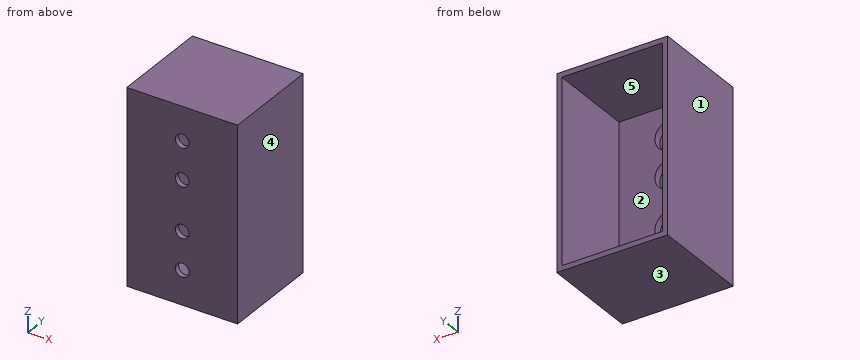
from build123d import *

# Parameters (mm, degrees)
EXTRUDE_1_DEPTH     = 73
SKETCH_2_W          = 44
SKETCH_2_H          = 39.5
EXTRUDE_2_DEPTH     = 2
SKETCH_3_W          = 44
SKETCH_3_H          = 39.5
EXTRUDE_3_DEPTH     = 2
SKETCH_4_R          = 2.75
CUT_EXTRUDE_1_DEPTH = 10
SKETCH_5_R          = 5.75
SKETCH_5_R_2        = 2.75
CUT_EXTRUDE_2_DEPTH = 3


with BuildPart() as part:
    # 草图1 → 凸台-拉伸1 (new body)
    with BuildSketch(Plane.XY):
        Polygon((-17.828125, 6.526041667), (-17.828125, -32.973958333), (26.171875, -32.973958333), (26.171875, 6.526041667), (24.171875, 6.526041667), (24.171875, -27.973958333), (-15.828125, -27.973958333), (-15.828125, 6.526041667), align=None)
    extrude(amount=EXTRUDE_1_DEPTH)

    # 草图2 → 凸台-拉伸2 (add)
    with BuildSketch(Plane.XY.offset(73)):
        with Locations((4.171875, -13.223958333)):
            Rectangle(SKETCH_2_W, SKETCH_2_H)
    extrude(amount=EXTRUDE_2_DEPTH)

    # 草图3 → 凸台-拉伸3 (add)
    with BuildSketch(Plane(origin=(0, 0, 0), x_dir=(-1, 0, 0), z_dir=(0, 0, -1))):
        with Locations((-4.171875, -13.223958333)):
            Rectangle(SKETCH_3_W, SKETCH_3_H)
    extrude(amount=EXTRUDE_3_DEPTH)

    # 草图4 → 切除-拉伸1 (cut)
    with BuildSketch(Plane(origin=(0, -27.973958333, 0), x_dir=(1, 0, 0), z_dir=(0, 1, 0))):
        with Locations(Location((4.171875, -26.5, 0), (0, 0, 180))):
            Circle(SKETCH_4_R)
        with Locations(Location((4.171875, -46.5, 0), (0, 0, 180))):
            Circle(SKETCH_4_R)
        with Locations(Location((4.171875, -11.5, 0), (0, 0, 180))):
            Circle(SKETCH_4_R)
        with Locations(Location((4.171875, -61.5, 0), (0, 0, 180))):
            Circle(SKETCH_4_R)
    extrude(amount=-CUT_EXTRUDE_1_DEPTH, mode=Mode.SUBTRACT)

    # 草图5 → 切除-拉伸2 (cut)
    # profile 1 of 4: a face of its own
    with BuildSketch(Plane(origin=(0, -27.973958333, 0), x_dir=(1, 0, 0), z_dir=(0, 1, 0))):
        with Locations(Location((4.171875, -61.5, 0), (0, 0, 180))):
            Circle(SKETCH_5_R)
        with Locations(Location((4.171875, -61.5, 0), (0, 0, 180))):
            Circle(SKETCH_5_R_2, mode=Mode.SUBTRACT)
    # profile 2 of 4: a face of its own
    with BuildSketch(Plane(origin=(0, -27.973958333, 0), x_dir=(1, 0, 0), z_dir=(0, 1, 0))):
        with Locations(Location((4.171875, -46.5, 0), (0, 0, 180))):
            Circle(SKETCH_5_R)
        with Locations(Location((4.171875, -46.5, 0), (0, 0, 180))):
            Circle(SKETCH_5_R_2, mode=Mode.SUBTRACT)
    # profile 3 of 4: a face of its own
    with BuildSketch(Plane(origin=(0, -27.973958333, 0), x_dir=(1, 0, 0), z_dir=(0, 1, 0))):
        with Locations(Location((4.171875, -26.5, 0), (0, 0, 180))):
            Circle(SKETCH_5_R)
        with Locations(Location((4.171875, -26.5, 0), (0, 0, 180))):
            Circle(SKETCH_5_R_2, mode=Mode.SUBTRACT)
    # profile 4 of 4: a face of its own
    with BuildSketch(Plane(origin=(0, -27.973958333, 0), x_dir=(1, 0, 0), z_dir=(0, 1, 0))):
        with Locations(Location((4.171875, -11.5, 0), (0, 0, 180))):
            Circle(SKETCH_5_R)
        with Locations(Location((4.171875, -11.5, 0), (0, 0, 180))):
            Circle(SKETCH_5_R_2, mode=Mode.SUBTRACT)
    extrude(amount=-CUT_EXTRUDE_2_DEPTH, mode=Mode.SUBTRACT)


solid = part.part
The listing builds one solid part. Answer for the finished solid, in the listing's coordinates (mm). Face numbers are marked on the shaded views. A direction names the side the tool comes from. Give positions to 0.01 mm unless a question says otherwise; leave off trailing zeros. Loops run counter-clockwise (first coordinate to the right, second up) from the corner with the lowest first, then second, coordinate; pieces in that order, holes last. Notation, with made-up numbers: (-35, -8) - (-8, -8) arc R30 ccw to (-8, 25) - close; hole circle Ø1 at (62, 29.25). An arc over 180 degrees is marked (long way). Use one line per item in the form item = value.
1. Find the intervals of material crossed by line 1 along Z through (x, y) = (16, -18); line 2 along X through (y, z) = (-12, 11); line 3 along Y through (x, z) = (22, 57), in increasing order. Write a range as [from, to].
Calculated:
line_1 = [-2, 0], [73, 75]
line_2 = [-17.83, -15.83], [24.17, 26.17]
line_3 = [-32.97, -27.97]
2. Section A-A on z = 26.5 is taken. Give the vertices of the cut face in (x, y), then the cut area to 4 significant figures.
Calculated:
outline = (-17.83, -32.97) - (1.42, -32.97) - (1.42, -30.97) - (-1.58, -30.97) - (-1.58, -27.97) - (-15.83, -27.97) - (-15.83, 6.53) - (-17.83, 6.53) - close; (6.92, -32.97) - (26.17, -32.97) - (26.17, 6.53) - (24.17, 6.53) - (24.17, -27.97) - (9.92, -27.97) - (9.92, -30.97) - (6.92, -30.97) - close
area = 312.5 mm^2
3. Given pin 1 Ø3.5 at (x, z) = (5, 44.5) entering from +Y; pin 2 Ø12.5 at (x, z) = (3, 10) entering from +Y; pin 3 Ø3.5 at (x, z) = (4.5, 62) entering from +Y, each flat-ended and moving along its own axis, determine where each tip first touches the part or whether it passes through.
Calculated:
pin_1 = -30.97
pin_2 = -27.97
pin_3 = through
4. Section C-C on x = 13 is taken. Give the vertices of the cut face in (y, z), then the cut area to 3 significant figures.
Calculated:
outline = (-32.97, -2) - (6.53, -2) - (6.53, 0) - (-27.97, 0) - (-27.97, 73) - (6.53, 73) - (6.53, 75) - (-32.97, 75) - close
area = 523 mm^2
5. Which of the six approach directions +Z, -Z, +X, -X, +Y, -Y give full straight-line access (tool end or side, diameter ignored) to the marked faces 4 and 5?
Calculated:
face_4 = +Z, -Z, +X, +Y, -Y
face_5 = +Y
6. Section B-B on y = -20 is taken. Give the vertices of the cut face in (x, z).
Calculated:
outline = (-17.83, -2) - (26.17, -2) - (26.17, 75) - (-17.83, 75) - close; hole (-15.83, 0) - (24.17, 0) - (24.17, 73) - (-15.83, 73) - close
7. The mould has two halves that part along X. Classify the marked faces 1, 2 and 3: pulls with the +X half, pulls with the -X half, needs draft (parallel to the pull), parting line crosses it, or undercut.
Calculated:
face_1 = pulls with the -X half
face_2 = undercut
face_3 = needs draft
